Geometry: final body of the model. Coordinates: model frame, mm. Round coordinates to 2 decimals unless told otherwise and drop trailing zeros. Loops run counter-clockwise (first coordinate to the right, second up) from the corner with the lowest first, then second, coordinate; pieces in that order, holes last. Notation, with made-up numbers: M 4.5,-35 L 63.5,-35 A9 cw 63.5,-23 Z; hole C 67,82.25 d2. An arc over 180 degrees is marked long. Answer as a JSON object with one key per item and string values.
```python
from build123d import *

# Parameters (mm, degrees)
CROQUIS1_W              = 511
CROQUIS1_H              = 705.8
SALIENTE_EXTRUIR1_DEPTH = 5
CROQUIS2_W              = 40
CROQUIS2_H              = 100
CORTAR_EXTRUIR1_DEPTH   = 10
CROQUIS4_W              = 110
CROQUIS4_H              = 98.950839499
CORTAR_EXTRUIR3_DEPTH   = 10
CROQUIS7_R              = 2.07
CORTAR_EXTRUIR6_DEPTH   = 10
CROQUIS8_R              = 2.07
CORTAR_EXTRUIR7_DEPTH   = 10


with BuildPart() as part:
    # Croquis1 → Saliente-Extruir1 (new body)
    with BuildSketch(Plane(origin=(0, 0, 0), x_dir=(1, 0, 0), z_dir=(0, 1, 0))):
        Rectangle(CROQUIS1_W, CROQUIS1_H)
    extrude(amount=SALIENTE_EXTRUIR1_DEPTH)

    # Croquis2 → Cortar-Extruir1 (cut)
    with BuildSketch(Plane(origin=(0, 0, 0), x_dir=(-1, 0, 0), z_dir=(0, -1, 0))):
        with Locations((235.5, -219.401276077)):
            Rectangle(CROQUIS2_W, CROQUIS2_H)
        with Locations((-235.5, -219.401276077)):
            Rectangle(CROQUIS2_W, CROQUIS2_H)
        with Locations((235.5, 0.598723923)):
            Rectangle(CROQUIS2_W, CROQUIS2_H)
        with Locations((-235.5, 0.598723923)):
            Rectangle(CROQUIS2_W, CROQUIS2_H)
    extrude(amount=-CORTAR_EXTRUIR1_DEPTH, mode=Mode.SUBTRACT)

    # Croquis4 → Cortar-Extruir3 (cut)
    with BuildSketch(Plane(origin=(0, 0, 0), x_dir=(-1, 0, 0), z_dir=(0, -1, 0))):
        with Locations((200.5, 211.875419749)):
            Rectangle(CROQUIS4_W, CROQUIS4_H)
        with Locations((-200.9, 211.875419749)):
            Rectangle(CROQUIS4_W, CROQUIS4_H)
    extrude(amount=-CORTAR_EXTRUIR3_DEPTH, mode=Mode.SUBTRACT)

    # Croquis7 → Cortar-Extruir6 (cut)
    with BuildSketch(Plane(origin=(0, 0, 0), x_dir=(-1, 0, 0), z_dir=(0, -1, 0))):
        with Locations(Location((236.6, -340.2, 0), (0, 0, 90))):
            Circle(CROQUIS7_R)
        with Locations(Location((211.2, -340.2, 0), (0, 0, 90))):
            Circle(CROQUIS7_R)
        with Locations(Location((185.8, -340.2, 0), (0, 0, 90))):
            Circle(CROQUIS7_R)
        with Locations(Location((160.4, -340.2, 0), (0, 0, 90))):
            Circle(CROQUIS7_R)
        with Locations(Location((135, -340.2, 0), (0, 0, 90))):
            Circle(CROQUIS7_R)
        with Locations(Location((109.6, -340.2, 0), (0, 0, 90))):
            Circle(CROQUIS7_R)
        with Locations(Location((84.2, -340.2, 0), (0, 0, 90))):
            Circle(CROQUIS7_R)
        with Locations(Location((58.8, -340.2, 0), (0, 0, 90))):
            Circle(CROQUIS7_R)
        with Locations(Location((33.4, -340.2, 0), (0, 0, 90))):
            Circle(CROQUIS7_R)
        with Locations(Location((8, -340.2, 0), (0, 0, 90))):
            Circle(CROQUIS7_R)
        with Locations(Location((-17.4, -340.2, 0), (0, 0, 90))):
            Circle(CROQUIS7_R)
        with Locations(Location((-42.8, -340.2, 0), (0, 0, 90))):
            Circle(CROQUIS7_R)
        with Locations(Location((-68.2, -340.2, 0), (0, 0, 90))):
            Circle(CROQUIS7_R)
        with Locations(Location((-93.6, -340.2, 0), (0, 0, 90))):
            Circle(CROQUIS7_R)
        with Locations(Location((-119, -340.2, 0), (0, 0, 90))):
            Circle(CROQUIS7_R)
        with Locations(Location((-144.4, -340.2, 0), (0, 0, 90))):
            Circle(CROQUIS7_R)
        with Locations(Location((-169.8, -340.2, 0), (0, 0, 90))):
            Circle(CROQUIS7_R)
        with Locations(Location((-195.2, -340.2, 0), (0, 0, 90))):
            Circle(CROQUIS7_R)
        with Locations(Location((-220.6, -340.2, 0), (0, 0, 90))):
            Circle(CROQUIS7_R)
        with Locations(Location((-246, -340.2, 0), (0, 0, 90))):
            Circle(CROQUIS7_R)
        with Locations(Location((242.8, -320.2, 0), (0, 0, 90))):
            Circle(CROQUIS7_R)
        with Locations(Location((242.8, -294.8, 0), (0, 0, 90))):
            Circle(CROQUIS7_R)
        with Locations(Location((242.8, -142.4, 0), (0, 0, 90))):
            Circle(CROQUIS7_R)
        with Locations(Location((242.8, -117, 0), (0, 0, 90))):
            Circle(CROQUIS7_R)
        with Locations(Location((242.8, -91.6, 0), (0, 0, 90))):
            Circle(CROQUIS7_R)
        with Locations(Location((242.8, -66.2, 0), (0, 0, 90))):
            Circle(CROQUIS7_R)
        with Locations(Location((242.8, 60.8, 0), (0, 0, 90))):
            Circle(CROQUIS7_R)
        with Locations(Location((242.8, 86.2, 0), (0, 0, 90))):
            Circle(CROQUIS7_R)
        with Locations(Location((242.8, 111.6, 0), (0, 0, 90))):
            Circle(CROQUIS7_R)
        with Locations(Location((242.8, 137, 0), (0, 0, 90))):
            Circle(CROQUIS7_R)
        with Locations(Location((242.8, 289.4, 0), (0, 0, 90))):
            Circle(CROQUIS7_R)
        with Locations(Location((242.8, 314.8, 0), (0, 0, 90))):
            Circle(CROQUIS7_R)
    extrude(amount=-CORTAR_EXTRUIR6_DEPTH, mode=Mode.SUBTRACT)

    # Croquis8 → Cortar-Extruir7 (cut)
    with BuildSketch(Plane(origin=(0, 0, 0), x_dir=(-1, 0, 0), z_dir=(0, -1, 0))):
        with Locations(Location((246, 340.2, 0), (0, 0, 90))):
            Circle(CROQUIS8_R)
        with Locations(Location((220.6, 340.2, 0), (0, 0, 90))):
            Circle(CROQUIS8_R)
        with Locations(Location((195.2, 340.2, 0), (0, 0, 90))):
            Circle(CROQUIS8_R)
        with Locations(Location((169.8, 340.2, 0), (0, 0, 90))):
            Circle(CROQUIS8_R)
        with Locations(Location((144.4, 340.2, 0), (0, 0, 90))):
            Circle(CROQUIS8_R)
        with Locations(Location((119, 340.2, 0), (0, 0, 90))):
            Circle(CROQUIS8_R)
        with Locations(Location((93.6, 340.2, 0), (0, 0, 90))):
            Circle(CROQUIS8_R)
        with Locations(Location((68.2, 340.2, 0), (0, 0, 90))):
            Circle(CROQUIS8_R)
        with Locations(Location((42.8, 340.2, 0), (0, 0, 90))):
            Circle(CROQUIS8_R)
        with Locations(Location((17.4, 340.2, 0), (0, 0, 90))):
            Circle(CROQUIS8_R)
        with Locations(Location((-8, 340.2, 0), (0, 0, 90))):
            Circle(CROQUIS8_R)
        with Locations(Location((-33.4, 340.2, 0), (0, 0, 90))):
            Circle(CROQUIS8_R)
        with Locations(Location((-58.8, 340.2, 0), (0, 0, 90))):
            Circle(CROQUIS8_R)
        with Locations(Location((-84.2, 340.2, 0), (0, 0, 90))):
            Circle(CROQUIS8_R)
        with Locations(Location((-109.6, 340.2, 0), (0, 0, 90))):
            Circle(CROQUIS8_R)
        with Locations(Location((-135, 340.2, 0), (0, 0, 90))):
            Circle(CROQUIS8_R)
        with Locations(Location((-160.4, 340.2, 0), (0, 0, 90))):
            Circle(CROQUIS8_R)
        with Locations(Location((-185.8, 340.2, 0), (0, 0, 90))):
            Circle(CROQUIS8_R)
        with Locations(Location((-211.2, 340.2, 0), (0, 0, 90))):
            Circle(CROQUIS8_R)
        with Locations(Location((-236.6, 340.2, 0), (0, 0, 90))):
            Circle(CROQUIS8_R)
        with Locations(Location((-242.8, 314.8, 0), (0, 0, 90))):
            Circle(CROQUIS8_R)
        with Locations(Location((-242.8, 289.4, 0), (0, 0, 90))):
            Circle(CROQUIS8_R)
        with Locations(Location((-242.8, 137, 0), (0, 0, 90))):
            Circle(CROQUIS8_R)
        with Locations(Location((-242.8, 111.6, 0), (0, 0, 90))):
            Circle(CROQUIS8_R)
        with Locations(Location((-242.8, 86.2, 0), (0, 0, 90))):
            Circle(CROQUIS8_R)
        with Locations(Location((-242.8, 60.8, 0), (0, 0, 90))):
            Circle(CROQUIS8_R)
        with Locations(Location((-242.8, -66.2, 0), (0, 0, 90))):
            Circle(CROQUIS8_R)
        with Locations(Location((-242.8, -91.6, 0), (0, 0, 90))):
            Circle(CROQUIS8_R)
        with Locations(Location((-242.8, -117, 0), (0, 0, 90))):
            Circle(CROQUIS8_R)
        with Locations(Location((-242.8, -142.4, 0), (0, 0, 90))):
            Circle(CROQUIS8_R)
        with Locations(Location((-242.8, -294.8, 0), (0, 0, 90))):
            Circle(CROQUIS8_R)
        with Locations(Location((-242.8, -320.2, 0), (0, 0, 90))):
            Circle(CROQUIS8_R)
    extrude(amount=-CORTAR_EXTRUIR7_DEPTH, mode=Mode.SUBTRACT)


solid = part.part
```
1) First-contact query: pin 1 (5 mm diameter, centred on x = -242.8, z = 142.4, fed in from -Y); pin 2 (3.5 mm diameter, centred on x = -135, z = 340.2, fed in from +Y); pin 3 (1 mm diameter, centred on y = 3, z = 188.5, fed in from +X). Flat tips, straight axial feed; report the tip coordinate or a pass-through.
Geometry results:
{"pin 1": "y = 0", "pin 2": "through", "pin 3": "x = 215.5"}
2) Cut plane A-A on z = -200.5. Return the cut outline in (x, y), and give its area (3 significant figures).
Geometry results:
{"outline": "M -145.5,0 L 145.9,0 L 145.9,5 L -145.5,5 Z", "area": "1,460 mm2"}
3) Cut plane C-C on z = -28.5. Return the cut outline in (x, y).
Geometry results:
{"outline": "M -215.5,0 L 215.5,0 L 215.5,5 L -215.5,5 Z"}
4) Line query: probe 1 along X at (y, z) = (0.3, 65.5); probe 2 along X at (y, z) = (4.5, 143); probe 3 along Z at (x, y) = (150.5, 3.15). Output: solid intervals per line, ascending.
Geometry results:
{"probe 1": "-255.5 to -244.75, -240.85 to 240.85, 244.75 to 255.5", "probe 2": "-255.5 to -244.78, -240.82 to 240.82, 244.78 to 255.5", "probe 3": "-352.9 to -261.35, -162.4 to 352.9"}
5) Cut plane B-B on y = 3.7. Count the separate pieces of the cut face and the enclosed holes in it, and give its area (3 significant figures).
Geometry results:
{"separate pieces": "1", "enclosed holes": "64", "area": "322,000 mm2"}
